For this review, take the finished solid that the model builds, in its own axes (mm). Give positions to 0.01 mm unless a question says otherwise; leave off trailing zeros. Loops run counter-clockwise (first coordinate to the right, second up) from the corner with the lowest first, then second, coordinate; pieces in that order, holes last. Notation, with made-up numbers: (71.5, 49) - (79.5, 49) arc R22 ccw to (79.5, 63) - close; hole circle Ø10 at (88, -1.75). An arc over 180 degrees is marked (long way). Put each result on its own line as item: value.
from build123d import *

# Parameters (mm, degrees)
F3_DEPTH = 12.001
F4_D     = 10.3


with BuildPart() as f2:
    # F1 (on Right) → F2 (revolve)
    with BuildSketch(Plane.YZ):
        Polygon((0, 9.5), (0, 0), (12, 0), (12, 7.4696551146), (8.5, 10.9696551146), (0, 10.9696551146), align=None)
    revolve(axis=Axis((0, 6, 0), (0, 1, 0)))

    # F0 (on Front) → F3 (cut, through all)
    with BuildSketch(Plane.XZ):
        with BuildLine():
            Line((-9.5, -5.4848275573), (-9.5, 0))
            Line((-9.5, 0), (-9.5, 5.4848275573))
            ThreePointArc((-9.5, 5.4848275573), (-10.9696551146, 0), (-9.5, -5.4848275573))
        make_face()
        with BuildLine():
            Line((-9.5, 5.4848275573), (-4.7499997625, 8.2272414731))
            Line((-4.7499997625, 8.2272414731), (0, 10.9696551146))
            ThreePointArc((0, 10.9696551146), (-5.4848275573, 9.5), (-9.5, 5.4848275573))
        make_face()
        with BuildLine():
            Line((0, 10.9696551146), (4.7499998306, 8.2272414337))
            Line((4.7499998306, 8.2272414337), (9.5, 5.4848275573))
            ThreePointArc((9.5, 5.4848275573), (5.4848275573, 9.5), (0, 10.9696551146))
        make_face()
        with BuildLine():
            Line((9.5, 5.4848275573), (9.5, 0))
            Line((9.5, 0), (9.5, -5.4848275573))
            ThreePointArc((9.5, -5.4848275573), (10.5958731807, -2.8391556619), (10.9696551146, 0))
            ThreePointArc((10.9696551146, 0), (10.5958731807, 2.8391556619), (9.5, 5.4848275573))
        make_face()
        with BuildLine():
            Line((9.5, -5.4848275573), (4.7499998306, -8.2272414337))
            Line((4.7499998306, -8.2272414337), (0, -10.9696551146))
            ThreePointArc((0, -10.9696551146), (5.4848275573, -9.5), (9.5, -5.4848275573))
        make_face()
        with BuildLine():
            Line((0, -10.9696551146), (-4.749999949, -8.2272413654))
            Line((-4.749999949, -8.2272413654), (-9.5, -5.4848275573))
            ThreePointArc((-9.5, -5.4848275573), (-5.4848275573, -9.5), (0, -10.9696551146))
        make_face()
    extrude(amount=-F3_DEPTH, mode=Mode.SUBTRACT)

    # F4 (through all)
    with Locations(Plane.XZ):
        with Locations((0, 0)):
            Hole(F4_D / 2)


solid = f2.part
1) Draft analysis for pull direction X (two halves, no side actions). For faces 1 (the face through (9.5, 5, 0)), 2 (the face through (2, 0, 5)), 3 (the face through (-4.91, 6.08, 1.55)), state which applies: pulls with the +X half, pulls with the -X half, needs draft (parallel to the pull), parting line crosses it, or undercut.
Geometry check:
face 1: pulls with the +X half
face 2: needs draft
face 3: undercut
2) Take a section at A-A on y = 2. State the section outline as (x, z) points, and give its area (3 significant figures).
Geometry check:
outline: (-9.5, -5.48) - (0, -10.97) - (9.5, -5.48) - (9.5, 5.48) - (0, 10.97) - (-9.5, 5.48) - close; hole circle Ø10.3 at (0, 0)
area: 229 mm²
3) Take a section at C-C on y = 9.5. State the section outline as (x, z) points.
Geometry check:
outline: (-9.5, -3.02) arc R9.97 ccw to (-7.37, -6.72) - (-2.13, -9.74) arc R9.97 ccw to (2.13, -9.74) - (7.37, -6.72) arc R9.97 ccw to (9.5, -3.02) - (9.5, 3.02) arc R9.97 ccw to (7.37, 6.72) - (2.13, 9.74) arc R9.97 ccw to (-2.13, 9.74) - (-7.37, 6.72) arc R9.97 ccw to (-9.5, 3.02) - close; hole circle Ø10.3 at (0, 0)
4) Insertion check: pin 1 Ø6 at (y, z) = (9.5, -8.5) entering from +X; pin 2 Ø6 at (x, z) = (-3, 3) entering from +Y; pin 3 Ø1.5 at (x, y) = (-4.5, 3) entering from +Z. Each pin has a flat end and moves straight along its axis. Give the tip position at first contact, or say it passes through.
Geometry check:
pin 1: stops at x = 9.25
pin 2: stops at y = 12
pin 3: stops at z = 8.8
5) Take a section at B-B on z = 0. State the section outline as (x, y) points.
Geometry check:
outline: (-9.5, 0) - (-5.15, 0) - (-5.15, 12) - (-7.47, 12) - (-9.5, 9.97) - close; (5.15, 0) - (9.5, 0) - (9.5, 9.97) - (7.47, 12) - (5.15, 12) - close
6) Wall thickness on line 1 (Z direction, x = -1, y = 11.25); line 2 (Z direction, x = 1.5, y = 9.75); line 3 (X direction, y = 8.5, z = -4.25): over which ranges is each line inside the solid? List them lowest first.
Geometry check:
line 1: z = -8.16 to -5.05, 5.05 to 8.16
line 2: z = -9.6 to -4.93, 4.93 to 9.6
line 3: x = -9.5 to -2.91, 2.91 to 9.5
